```python
from build123d import *

# Parameters (mm, degrees)
SKETCH1_R           = 25
BOSS_EXTRUDE1_DEPTH = 30
SKETCH2_OUTSIDE_W   = 67.362
SKETCH2_OUTSIDE_H   = 67.362
SKETCH2_OUTSIDE_R   = 19.25
CUT_EXTRUDE1_DEPTH  = 25
SKETCH3_R           = 16
CUT_EXTRUDE2_DEPTH  = 9
SKETCH4_R           = 10.5
CUT_EXTRUDE3_DEPTH  = 22
SKETCH5_R           = 16
CUT_EXTRUDE4_DEPTH  = 18


with BuildPart() as part:
    # Sketch1 → Boss-Extrude1 (new body)
    with BuildSketch(Plane(origin=(0, 0, 0), x_dir=(1, 0, 0), z_dir=(0, 1, 0))):
        Circle(SKETCH1_R)
    extrude(amount=BOSS_EXTRUDE1_DEPTH)

    # Sketch2 outside → Cut-Extrude1 (cut)
    with BuildSketch(Plane(origin=(0, 30, 0), x_dir=(1, 0, 0), z_dir=(0, 1, 0))):
        Rectangle(SKETCH2_OUTSIDE_W, SKETCH2_OUTSIDE_H)
        Circle(SKETCH2_OUTSIDE_R, mode=Mode.SUBTRACT)
    extrude(amount=-CUT_EXTRUDE1_DEPTH, mode=Mode.SUBTRACT)

    # Sketch3 → Cut-Extrude2 (cut)
    with BuildSketch(Plane(origin=(0, 30, 0), x_dir=(1, 0, 0), z_dir=(0, 1, 0))):
        Circle(SKETCH3_R)
    extrude(amount=-CUT_EXTRUDE2_DEPTH, mode=Mode.SUBTRACT)

    # Sketch4 → Cut-Extrude3 (cut, through all)
    with BuildSketch(Plane(origin=(0, 21, 0), x_dir=(1, 0, 0), z_dir=(0, 1, 0))):
        Circle(SKETCH4_R)
    extrude(amount=-CUT_EXTRUDE3_DEPTH, mode=Mode.SUBTRACT)

    # Sketch5 → Cut-Extrude4 (cut)
    with BuildSketch(Plane.XZ):
        Circle(SKETCH5_R)
    extrude(amount=-CUT_EXTRUDE4_DEPTH, mode=Mode.SUBTRACT)


solid = part.part
```
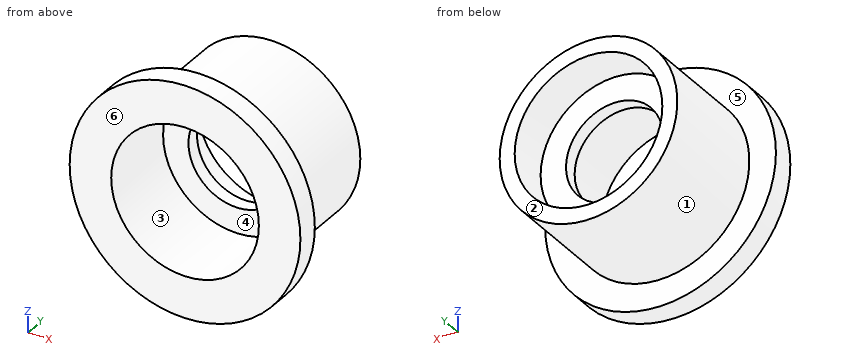
Check sheet for the modelled part. Datum: model origin and axes. Units: mm. Face numbers are marked on the shaded views. A direction names the side the tool comes from. Give positions to 0.01 mm unless a question says otherwise; leave off trailing zeros. Write each loop counter-clockwise with the first axis right and the second up, starting at its lowest first coordinate (ties: lowest second). Pieces come first, ordered by that corner, then holes. Notation, with made-up numbers: (-27, 23.5) - (-11, 23.5) arc R18 ccw to (-11, 55.5) - close; hole circle Ø7 at (27, 29.25). An arc over 180 degrees is marked (long way). Answer as a JSON object with one key per item and string values. Group by question number.
1) Sectioned sample at A-A (z = 0). Record the cut outline in (x, y).
2) Sectioned sample at C-C (y = 6). Record the cut outline in (x, z), then the cut area to 3 significant figures.
3) Release check for a two-part mould opening along X. For the marked faces 1, 2, 3 and 4 record: pulls with the +X half, pulls with the -X half, needs draft (parallel to the pull), parting line crosses it, or undercut.
4) Thickness scan on probe 1 along X at (y, z) = (26.5, 0); probe 2 along Z at (x, y) = (0, 20.4). Record the ranges inside material, lowest first. Write a range as from..to.
5) Sectioned sample at B-B (x = 0). Record the cut outline in (y, z).
6) Access from +Z, -Z, +X, -X, +Y, -Y to the whole of each face (thin tool, end or side, straight path). Record for the marked faces 5 and 6.
7) Sectioned sample at D-D (x = 18.5). Record the cut outline in (y, z), then the cut area to 3 significant figures.
8) Depth check by flat-ended pin: P1, Ø3, axis at y = 24.5, z = 4, coming from the -X side; P2, Ø1, axis at x = 4, y = 15, coming from the +Z side; P3, Ø10, axis at y = 25.5, z = -6.5, coming from the +X side. Enter the tip coordinate at first touch or a pass-through.
Geometry results:
{
 "1": {"outline": "(-25, 0) - (-16, 0) - (-16, 18) - (-10.5, 18) - (-10.5, 21) - (-16, 21) - (-16, 30) - (-19.25, 30) - (-19.25, 5) - (-25, 5) - close; (10.5, 18) - (16, 18) - (16, 0) - (25, 0) - (25, 5) - (19.25, 5) - (19.25, 30) - (16, 30) - (16, 21) - (10.5, 21) - close"},
 "2": {"outline": "circle Ø38.5 at (0, 0); hole circle Ø32 at (0, 0)", "area": "360 mm^2"},
 "3": {"face 1": "parting line crosses it", "face 2": "needs draft", "face 3": "undercut", "face 4": "undercut"},
 "4": {"probe 1": "x = -19.25..-16, 16..19.25", "probe 2": "z = -19.25..-10.5, 10.5..19.25"},
 "5": {"outline": "(0, -25) - (5, -25) - (5, -19.25) - (30, -19.25) - (30, -16) - (21, -16) - (21, -10.5) - (18, -10.5) - (18, -16) - (0, -16) - close; (0, 16) - (18, 16) - (18, 10.5) - (21, 10.5) - (21, 16) - (30, 16) - (30, 19.25) - (5, 19.25) - (5, 25) - (0, 25) - close"},
 "6": {"face 5": "+Y", "face 6": "+Z, -Z, +X, -X, -Y"},
 "7": {"outline": "(0, -16.82) - (5, -16.82) - (5, -5.32) - (30, -5.32) - (30, 5.32) - (5, 5.32) - (5, 16.82) - (0, 16.82) - close", "area": "434 mm^2"},
 "8": {"P1": "stops at x = -19.09", "P2": "stops at z = 18.93", "P3": "stops at x = 19.19"}
}
